```python
from build123d import *

# Parameters (mm, degrees)
CYLINDER002_R       = 13.5
CYLINDER002_DEPTH   = 2
CYLINDER001_R       = 18
CYLINDER001_DEPTH   = 2
CUT_PLACEMENT_ANGLE = 180


with BuildPart() as cylinder002:
    # Cylinder002 → Cylinder002 (new body)
    with BuildSketch(Plane.XY):
        Circle(CYLINDER002_R)
    extrude(amount=CYLINDER002_DEPTH)


with BuildPart() as base:
    # Cylinder001 → Cylinder001 (new body)
    with BuildSketch(Plane.XY):
        Circle(CYLINDER001_R)
    extrude(amount=CYLINDER001_DEPTH)

    # Cut: cut Cylinder002
    add(cylinder002.part, mode=Mode.SUBTRACT)


with BuildPart() as base_1:
    # Cut placement: moved
    add(base.part.moved(Location((0, 0, 2))).rotate(Axis((0, 0, 2), (1, 0, 0)), CUT_PLACEMENT_ANGLE))


solid = base_1.part
```
Verification items for the finished model (mm, model axes). Round coordinates to 2 decimals unless told otherwise and drop trailing zeros. Write each loop counter-clockwise with the first axis right and the second up, starting at its lowest first coordinate (ties: lowest second). Pieces come first, ordered by that corner, then holes. Notation, with made-up numbers: (51.5, 63) - (100.5, 63) arc R12 cw to (100.5, 69) - close; hole circle Ø1 at (80.5, 74.5). An arc over 180 degrees is marked (long way). Answer as a JSON object with one key per item and string values. Group by question number.
Q1. Thickness scan on line 1 (Y direction, x = 0, z = 1.3); line 2 (Y direction, x = -8, z = 1.5). Record the ranges inside material, lowest first.
Q2. Section check A-A, the plane y = 0. Enter the section's corners in (x, z).
Q3. Section check D-D, the plane x = 14.5. Enter the section's corners in (y, z).
Q4. Mould release check, pull along X, two halves, no side actions. Record for faces 1 (the cylindrical face through (-2.93, 13.18, 1.01)), 2 (the flat face through (2.58, -13.42, 2)), 3 (the cylindrical face through (-2.343, -17.847, 1.014)): released by +X, released by -X, zero draft, split by the parting line, or undercut.
Q5. Section check C-C, the plane z = 0.75. Enter the section's corners in (x, y), plus the area to 3 significant figures.
Found:
{
 "1": {"line 1": "y = -18 to -13.5, 13.5 to 18", "line 2": "y = -16.12 to -10.87, 10.87 to 16.12"},
 "2": {"outline": "(-18, 0) - (-13.5, 0) - (-13.5, 2) - (-18, 2) - close; (13.5, 0) - (18, 0) - (18, 2) - (13.5, 2) - close"},
 "3": {"outline": "(-10.67, 0) - (10.67, 0) - (10.67, 2) - (-10.67, 2) - close"},
 "4": {"face 1": "undercut", "face 2": "zero draft", "face 3": "split by the parting line"},
 "5": {"outline": "circle Ø36 at (0, 0); hole circle Ø27 at (0, 0)", "area": "445 mm^2"}
}
